Here's how the part is built. I have some questions about the finished solid (model axes, mm). A direction names the side the tool comes from. Round coordinates to 2 decimals unless told otherwise and drop trailing zeros. Loops run counter-clockwise (first coordinate to the right, second up) from the corner with the lowest first, then second, coordinate; pieces in that order, holes last. Notation, with made-up numbers: M 78,44 L 91,44 A20 cw 91,67 Z; hole C 50,67 d8. An arc over 180 degrees is marked long. Put each result on its own line as item: value. Start each with the question number.
```python
from build123d import *

# Parameters (mm, degrees)
SKETCH_2_R          = 1
SKETCH_2_W          = 12
SKETCH_2_H          = 10
EXTRUDE_1_DEPTH     = 3
SKETCH_3_W          = 67.5
SKETCH_3_H          = 19.05
CUT_EXTRUDE_1_DEPTH = 3
SKETCH_4_W          = 6
SKETCH_4_H          = 3
CUT_EXTRUDE_2_DEPTH = 3
CUT_EXTRUDE_START   = -3
CUT_EXTRUDE_3_DEPTH = 3


with BuildPart() as part:
    # 스케치2 → 보스-돌출1 (new body)
    with BuildSketch(Plane.XY):
        with BuildLine():
            Line((-25.485574715, -6.758293196), (31.501216284, -6.758293196))
            ThreePointArc((31.501216284, -6.758293196), (38.452055955, -4.004295945), (41.630451907, 2.763013133))
            ThreePointArc((41.630451907, 2.763013133), (34.930270172, 4.650120348), (27.980151111, 4.263527588))
            ThreePointArc((27.980151111, 4.263527588), (30.476148958, 15.174416231), (26.885608279, 25.775619647))
            ThreePointArc((26.885608279, 25.775619647), (19.196067088, 24.921345998), (12.532472084, 20.9900194))
            ThreePointArc((12.532472084, 20.9900194), (7.013386949, 25.131320034), (0.635, 27.763211294))
            ThreePointArc((0.635, 27.763211294), (-5.803216647, 23.07550321), (-10.623464465, 16.735909244))
            ThreePointArc((-10.623464465, 16.735909244), (-16.694266299, 18.270908366), (-22.954465563, 18.415))
            ThreePointArc((-22.954465563, 18.415), (-24.716513625, 12.803357438), (-25.333146618, 6.95398915))
            ThreePointArc((-25.333146618, 6.95398915), (-32.051736926, 6.951939733), (-37.86649166, 3.586217327))
            ThreePointArc((-37.86649166, 3.586217327), (-33.552420479, -3.831808304), (-25.485574715, -6.758293196))
        make_face()
        with Locations((-18.720080529, 13.97)):
            Circle(SKETCH_2_R, mode=Mode.SUBTRACT)
        with Locations((0.635, 22.758099244)):
            Circle(SKETCH_2_R, mode=Mode.SUBTRACT)
        with Locations((24.024354369, 20.291387406)):
            Circle(SKETCH_2_R, mode=Mode.SUBTRACT)
        with Locations((3.600778132, 11.95398915)):
            Rectangle(SKETCH_2_W, SKETCH_2_H, mode=Mode.SUBTRACT)
    extrude(amount=EXTRUDE_1_DEPTH)

    # 스케치3 → 컷-돌출1 (cut)
    with BuildSketch(Plane.XY.offset(3)):
        with Locations((0.583193505, -10.568293196)):
            Rectangle(SKETCH_3_W, SKETCH_3_H)
    extrude(amount=-CUT_EXTRUDE_1_DEPTH, mode=Mode.SUBTRACT)

    # 스케치4 → 컷-돌출2 (cut)
    with BuildSketch(Plane.XY.offset(3)):
        with Locations((-20.006806495, 0.456706804)):
            Rectangle(SKETCH_4_W, SKETCH_4_H)
        with Locations((17.393193505, 0.456706804)):
            Rectangle(SKETCH_4_W, SKETCH_4_H)
        with Locations((-1.306806495, 0.456706804)):
            Rectangle(SKETCH_4_W, SKETCH_4_H)
    extrude(amount=-CUT_EXTRUDE_2_DEPTH, mode=Mode.SUBTRACT)

    # 스케치6 → 컷-돌출3 (cut)
    with BuildSketch(Plane.XY.offset(3).offset(CUT_EXTRUDE_START)):
        with BuildLine():
            Line((-17.006806495, 1.956706804), (-23.006806495, 1.956706804))
            Line((-23.006806495, 1.956706804), (-23.006806495, -1.043293196))
            Line((-23.006806495, -1.043293196), (-33.166806495, -1.043293196))
            Line((-33.166806495, -1.043293196), (-33.166806495, -4.141334476))
            ThreePointArc((-33.166806495, -4.141334476), (-36.235049915, -0.71447027), (-37.86649166, 3.586217327))
            ThreePointArc((-37.86649166, 3.586217327), (-32.051736926, 6.951939733), (-25.333146618, 6.95398915))
            ThreePointArc((-25.333146618, 6.95398915), (-24.716513625, 12.803357438), (-22.954465563, 18.415))
            ThreePointArc((-22.954465563, 18.415), (-16.694266299, 18.270908366), (-10.623464465, 16.735909244))
            ThreePointArc((-10.623464465, 16.735909244), (-5.803216647, 23.07550321), (0.635, 27.763211294))
            ThreePointArc((0.635, 27.763211294), (7.013386949, 25.131320034), (12.532472084, 20.9900194))
            ThreePointArc((12.532472084, 20.9900194), (19.196067088, 24.921345998), (26.885608279, 25.775619647))
            ThreePointArc((26.885608279, 25.775619647), (30.476148958, 15.174416231), (27.980151111, 4.263527588))
            ThreePointArc((27.980151111, 4.263527588), (34.930270172, 4.650120348), (41.630451907, 2.763013133))
            ThreePointArc((41.630451907, 2.763013133), (39.424820657, -2.950900295), (34.333193505, -6.355154812))
            Line((34.333193505, -6.355154812), (34.333193505, -1.043293196))
            Line((34.333193505, -1.043293196), (34.333193505, 1.956706804))
            Line((34.333193505, 1.956706804), (28.736134873, 1.956706804))
            ThreePointArc((28.736134873, 1.956706804), (21.761064735, 6.755645136), (23.749798637, 14.985247192))
            ThreePointArc((23.749798637, 14.985247192), (24.996231791, 16.035094284), (26.305425054, 17.005551662))
            ThreePointArc((26.305425054, 17.005551662), (26.732453483, 23.235228296), (20.559975673, 22.290907411))
            ThreePointArc((20.559975673, 22.290907411), (11.947819263, 17.903967637), (4.440273192, 23.99093984))
            ThreePointArc((4.440273192, 23.99093984), (-0.484844776, 26.598144514), (-3.236462793, 21.752228554))
            ThreePointArc((-3.236462793, 21.752228554), (-6.999770707, 13.865014257), (-15.414747401, 16.222725663))
            ThreePointArc((-15.414747401, 16.222725663), (-20.472957028, 17.565472706), (-22.530630542, 12.753567266))
            ThreePointArc((-22.530630542, 12.753567266), (-20.728909441, 10.511010783), (-17.88821468, 10.057456172))
            ThreePointArc((-17.88821468, 10.057456172), (-13.029100566, 6.902297391), (-16.184259346, 2.043183277))
            ThreePointArc((-16.184259346, 2.043183277), (-16.593266293, 1.978385333), (-17.006806495, 1.956706804))
        make_face()
    extrude(amount=CUT_EXTRUDE_3_DEPTH, mode=Mode.SUBTRACT)


solid = part.part
```
1) I'm going to push flat-ended pins straight in: P1, Ø0.9, axis at y = 1, z = 2, coming from the -X side; P2, Ø1.5, axis at x = 18, z = 1.5, coming from the -Y side; P3, Ø1, axis at y = 12.5, z = 1.5, coming from the +X side. Where does each tip first touch, or does it pass through?
2) If we mould it in two halves opening along X, with no side actions, what happens to faces 1 (the face through (1.693, 0, 2)), 2 (the face through (5, 4, 3)), 3 (the face through (-17.007, 0, 2)), 4 (the face through (17, 1.957, 2))? For each: pulls with the +X half, pulls with the -X half, needs draft (parallel to the pull), parting line crosses it, or undercut.
3) Suppose I cut it at B-B (x = 7). Write out the boundary of the cut face in (y, z), plus the area to 3 significant figures.
4) On a 3-axis mill with a long thin cutter (end or side, diameter ignored), from which of +Z, -Z, +X, -X, +Y, -Y can I reach the whole of each face in a straight line? I mean faces 5 (the face through (34.333, 0, 1)), 6 (the face through (9.601, 12, 1)), 7 (the face through (-1, 1.957, 2)). Say none if no direction works.
5) Suppose I cut it at D-D (x = 27). Write out the boundary of the cut face in (y, z).
6) Suppose I cut it at C-C (z = 1.25). Write out the boundary of the cut face in (x, y) (3 decimals).
7) Suppose I cut it at A-A (y = 13.97). Write out the boundary of the cut face in (x, z).
8) If I drill on probe 1 along X at (y, z) = (9.5, 2.45); probe 2 along Y at (x, z) = (25.5, 1.15); probe 3 along Y at (x, z) = (30, 0.65), over which ranges is the centre line in solid material (lowest first)? Write a range as from..to.
Results are:
1. P1: x = -17.01
1. P2: y = 1.96
1. P3: x = 22.18
2. face 1: undercut
2. face 2: needs draft
2. face 3: pulls with the -X half
2. face 4: undercut
3. outline: M -1.04,0 L 6.95,0 L 6.95,3 L -1.04,3 Z; M 16.95,0 L 20.08,0 L 20.08,3 L 16.95,3 Z
3. area: 33.4 mm²
4. face 5: +Z, -Z, +X, +Y, -Y
4. face 6: +Z, -Z
4. face 7: +Z, -Z, -Y
5. outline: M -1.04,0 L 2.16,0 L 2.16,3 L -1.04,3 Z; M 17.62,0 L 22.96,0 L 22.96,3 L 17.62,3 Z
6. outline: M -17.888,10.057 A4.097 cw -16.184,2.043 A3.955 cw -17.007,1.957 L -17.007,-1.043 L -4.307,-1.043 L -4.307,1.957 L 1.693,1.957 L 1.693,-1.043 L 14.393,-1.043 L 14.393,1.957 L 20.393,1.957 L 20.393,-1.043 L 34.333,-1.043 L 34.333,1.957 L 28.736,1.957 A7.468 cw 23.75,14.985 A26.243 cw 26.305,17.006 A4 ccw long 20.56,22.291 A8.87 cw 4.44,23.991 A4 ccw -3.236,21.752 A6.788 cw -15.415,16.223 A4 ccw long Z; hole C -18.72,13.97 d2; hole M -2.399,6.954 L 9.601,6.954 L 9.601,16.954 L -2.399,16.954 Z; hole C 0.635,22.758 d2; hole C 24.024,20.291 d2
7. outline: M -22.72,0 L -19.72,0 L -19.72,3 L -22.72,3 Z; M -17.72,0 L -12.83,0 L -12.83,3 L -17.72,3 Z; M -6.78,0 L -2.4,0 L -2.4,3 L -6.78,3 Z; M 9.6,0 L 22.81,0 L 22.81,3 L 9.6,3 Z
8. probe 1: -14.83..-2.4, 9.6..21.27
8. probe 2: -1.04..2.69, 16.42..24.01
8. probe 3: -1.04..1.96
